Build history of the part. All positions in model axes, mm. A direction names the side the tool comes from. Coordinates: 2 decimals unless noted, no trailing zeros. Write each loop counter-clockwise with the first axis right and the second up, starting at its lowest first coordinate (ties: lowest second). Pieces come first, ordered by that corner, then holes.
from build123d import *

# Parameters (mm, degrees)
F1_DEPTH    = 9.144
F3_DEPTH    = 2.794
F5_DEPTH    = 3.2766
F6_T1_DEPTH = 12.7
F6_T4_ANGLE = 180
F6_T6_ANGLE = 180
F7_R        = 5.08


# Not quite as in the source:
# - a fillet or chamfer that OpenCascade refuses, or shapes differently, is made with other operations: its cross-section is extruded or revolved along the edge and cut away or added


with BuildPart() as f1:
    # F0 (on Front) → F1 (new body)
    with BuildSketch(Plane.XZ):
        with BuildLine():
            Line((12.7, 12.7), (0, 12.7))
            ThreePointArc((0, 12.7), (-6.35, 6.35), (0, 0))
            Line((0, 0), (12.7, 0))
            ThreePointArc((12.7, 0), (19.05, 6.35), (12.7, 12.7))
        make_face()
    extrude(amount=F1_DEPTH)

    # F2 (on face) → F3 (join)
    with BuildSketch(Plane(origin=(0, 0, 0), x_dir=(-1, 0, 0), z_dir=(0, 1, 0))):
        with BuildLine():
            ThreePointArc((0, 2.032), (4.318, 6.35), (0, 10.668))
            Line((0, 10.668), (-12.7, 10.668))
            ThreePointArc((-12.7, 10.668), (-17.018, 6.35), (-12.7, 2.032))
            Line((-12.7, 2.032), (0, 2.032))
        make_face()
    extrude(amount=F3_DEPTH)

    # F4 (on face) → F5 (join)
    with BuildSketch(Plane(origin=(0, 2.794, 0), x_dir=(-1, 0, 0), z_dir=(0, 1, 0))):
        with BuildLine():
            Line((-12.7, 1.524), (0, 1.524))
            ThreePointArc((0, 1.524), (4.826, 6.35), (0, 11.176))
            Line((0, 11.176), (-12.7, 11.176))
            ThreePointArc((-12.7, 11.176), (-17.526, 6.35), (-12.7, 1.524))
        make_face()
    extrude(amount=F5_DEPTH)

    # F6: fillet of radius 5.08 on 4 edges, made by hand

    # F6_s2 → F6_t1 (cut)
    with BuildSketch(Plane.YZ):
        with BuildLine():
            ThreePointArc((2.794, 11.176), (5.1719677188, 9.3117646326), (6.0706, 6.4268791929))
            Line((6.0706, 6.4268791929), (6.0706, 11.176))
            Line((6.0706, 11.176), (2.794, 11.176))
        make_face()
        with BuildLine():
            ThreePointArc((2.794, 1.524), (5.1719677188, 3.3882353674), (6.0706, 6.2731208071))
            Line((6.0706, 6.2731208071), (6.0706, 1.524))
            Line((6.0706, 1.524), (2.794, 1.524))
        make_face()
    extrude(amount=F6_T1_DEPTH, mode=Mode.SUBTRACT)

    # F6_s3 → F6_t4 (revolve, cut)
    with BuildSketch(Plane.YZ.offset(12.7)):
        with BuildLine():
            ThreePointArc((2.794, 11.176), (5.1719677188, 9.3117646326), (6.0706, 6.4268791929))
            Line((6.0706, 6.4268791929), (6.0706, 11.176))
            Line((6.0706, 11.176), (2.794, 11.176))
        make_face()
    revolve(axis=Axis((12.7, 6.0706, 6.35), (0, 1, 0)), revolution_arc=F6_T4_ANGLE, mode=Mode.SUBTRACT)

    # F6_s5 → F6_t6 (revolve, cut)
    with BuildSketch(Plane.YZ):
        with BuildLine():
            ThreePointArc((6.0706, 6.2731208071), (5.1719677188, 3.3882353674), (2.794, 1.524))
            Line((2.794, 1.524), (6.0706, 1.524))
            Line((6.0706, 1.524), (6.0706, 6.2731208071))
        make_face()
    revolve(axis=Axis((0, 6.0706, 6.35), (0, 1, 0)), revolution_arc=F6_T6_ANGLE, mode=Mode.SUBTRACT)

    # F7
    f7_edges = [f1.edges().sort_by_distance(p)[0] for p in [
        (6.35, -9.144, 12.7),
        (19.05, -9.144, 6.35),
        (6.35, -9.144, 0),
        (-6.35, -9.144, 6.35),
    ]]
    fillet(f7_edges, radius=F7_R)


solid = f1.part
(1) Two-plate mould, pull along Y, no slides. Class faces 4 (the cylindrical face through (6.261, 5.147, 3.353)), 5 (the flat face through (6, 1, 10.668)), 6 (the flat face through (6, -9.144, 6)): pulls with the +Y half, pulls with the -Y half, needs draft (parallel to the pull), parting line crosses it, or undercut.
(2) Flat gauge pins, fed straight in: P1, Ø0.8, axis at x = 4.5, y = 1.5, coming from the -Z side; P2, Ø4, axis at x = 11.5, y = 4, coming from the +Z side; P3, Ø2, axis at x = 9, y = -7, coming from the -Z side. Where does each tip first touch, or does it go through?
(3) 3-axis set-ups, long thin cutter, end or side, ignore diameter. For faces 1 (the cylindrical face through (17.017, 1.377, 6.445)), 2 (the flat face through (6, 2.794, 11)), 3 (the cylindrical face through (-4.317, 1.377, 6.255)): which of +Z, -Z, +X, -X, +Y, -Y reach the whole face in a straight line?
(4) Probe L1, parallel to X at y = 1, z = 6.5; L2, parallel to Y at x = 16.5, z = 9; L3, parallel to X at y = 4.25, z = 6. List the from-to ranges inside material, lowest first.
(5) Slice it at A-A, the plane x = 1. List the corners of the cut face in (y, z), and give its area (3 significant figures).
(6) Slice it at B-B, the plane y = 2.25. List the corners of the cut face in (x, z).
(7) Slice it at C-C, the plane y = -1.75. List the corners of the cut face in (x, z), and give its area (3 significant figures).
Results:
1. face 4: pulls with the +Y half
1. face 5: undercut
1. face 6: pulls with the -Y half
2. P1: stops at z = 2.03
2. P2: stops at z = 11.18
2. P3: stops at z = 0.38
3. face 1: +X
3. face 2: none
3. face 3: -X
4. L1: x = -4.32 to 17.02
4. L2: y = -7.87 to 0, 2.79 to 3.24
4. L3: x = -3.96 to 16.66
5. outline: (-9.14, 5.08) arc R5.08 ccw to (-4.06, 0) - (0, 0) - (0, 2.03) - (2.79, 2.03) - (2.79, 1.52) arc R5.08 ccw to (6.07, 6.27) - (6.07, 6.43) arc R5.08 ccw to (2.79, 11.18) - (2.79, 10.67) - (0, 10.67) - (0, 12.7) - (-4.06, 12.7) arc R5.08 ccw to (-9.14, 7.62) - close
5. area: 152 mm2
6. outline: (0, 2.03) - (12.7, 2.03) arc R4.32 ccw to (12.7, 10.67) - (0, 10.67) arc R4.32 ccw to start
7. outline: (0, 0) - (12.7, 0) arc R6.35 ccw to (12.7, 12.7) - (0, 12.7) arc R6.35 ccw to start
7. area: 288 mm2
